from build123d import *

# Parameters (mm, degrees)
SKETCH1_W           = 36
SKETCH1_H           = 36
BOSS_EXTRUDE1_DEPTH = 186.9
FILLET1_SIZE        = 24
SKETCH2_R           = 2
CUT_EXTRUDE1_DEPTH  = 5
SKETCH3_W           = 4.8
SKETCH3_H           = 4.8
BOSS_EXTRUDE2_DEPTH = 4
SKETCH4_W           = 6
SKETCH4_H           = 4
CUT_EXTRUDE2_DEPTH  = 9
SKETCH5_W           = 3
SKETCH5_H           = 3
SKETCH5_W_2         = 12
SKETCH5_H_2         = 12
CUT_EXTRUDE3_DEPTH  = 10
SKETCH6_W           = 9
SKETCH6_H           = 6
CUT_EXTRUDE4_DEPTH  = 2


with BuildPart() as part:
    # Sketch1 → Boss-Extrude1 (new body)
    with BuildSketch(Plane(origin=(0, 0, 0), x_dir=(1, 0, 0), z_dir=(0, 1, 0))):
        with Locations((18, 18)):
            Rectangle(SKETCH1_W, SKETCH1_H)
    extrude(amount=BOSS_EXTRUDE1_DEPTH)

    # Fillet1
    # a fillet whose section is not a circle: 24 mm, written as the material it takes off along each edge
    with BuildSketch(Plane(origin=(0, -60, 0), x_dir=(1, 0, 0), z_dir=(0, 1, 0))) as fillet1_piece_1:
        with BuildLine():
            Bezier((FILLET1_SIZE, 0), (0, 0), (0, FILLET1_SIZE), weights=[1, 1.222222222, 1])
            Line((0, FILLET1_SIZE), (0, 0))
            Line((0, 0), (FILLET1_SIZE, 0))
        make_face()
    extrude(amount=306.9, mode=Mode.SUBTRACT)

    # Sketch2 → Cut-Extrude1 (cut)
    with BuildSketch(Plane.XZ):
        with Locations(Location((18, -18, 0), (0, 0, 270))):
            Circle(SKETCH2_R)
    extrude(amount=-CUT_EXTRUDE1_DEPTH, mode=Mode.SUBTRACT)

    # Sketch3 → Boss-Extrude2 (add)
    with BuildSketch(Plane.XZ):
        Polygon((26.2, -5), (31, -5), (31, -31), (26, -31), (5, -31), (5, -26.2), (26.2, -26.2), align=None)
        with Locations((11.8, -11.8)):
            Rectangle(SKETCH3_W, SKETCH3_H)
    extrude(amount=BOSS_EXTRUDE2_DEPTH)

    # Sketch4 → Cut-Extrude2 (cut)
    with BuildSketch(Plane(origin=(0, 0, -36), x_dir=(-1, 0, 0), z_dir=(0, 0, -1))):
        with Locations((-7, 180.9)):
            Rectangle(SKETCH4_W, SKETCH4_H)
        with Locations((-29, 180.9)):
            Rectangle(SKETCH4_W, SKETCH4_H)
        with Locations((-7, 160.9)):
            Rectangle(SKETCH4_W, SKETCH4_H)
    extrude(amount=-CUT_EXTRUDE2_DEPTH, mode=Mode.SUBTRACT)

    # Sketch5 → Cut-Extrude3 (cut)
    with BuildSketch(Plane(origin=(0, 186.9, 0), x_dir=(1, 0, 0), z_dir=(0, 1, 0))):
        with Locations((7, 31.5)):
            Rectangle(SKETCH5_W, SKETCH5_H)
        with Locations((18, 18)):
            Rectangle(SKETCH5_W_2, SKETCH5_H_2)
    extrude(amount=-CUT_EXTRUDE3_DEPTH, mode=Mode.SUBTRACT)

    # Sketch6 → Cut-Extrude4 (cut)
    with BuildSketch(Plane(origin=(0, 186.9, 0), x_dir=(1, 0, 0), z_dir=(0, 1, 0))):
        with Locations((7, 30)):
            Rectangle(SKETCH6_W, SKETCH6_H)
    extrude(amount=-CUT_EXTRUDE4_DEPTH, mode=Mode.SUBTRACT)


solid = part.part
Work out the finished part from the listing and answer in its coordinate system (mm). A direction names the side the tool comes from. Give positions to 0.01 mm unless a question says otherwise; leave off trailing zeros. Answer in a Markdown table with one row per item. Add a question column.
Q1. Determine the mould class of faces 1 (the flat face through (10, 181, -32)), 2 (the cylindrical face through (20, 2, -18)), 3 (the flat face through (12, -2, -9.4)) for opening direction Z: released by +Z, released by -Z, zero draft, split by the parting line, or undercut.
Q2. Consider line 1 along X through (y, z) = (177.5, -22); line 2 along Y through (x, z) = (33, -5); line 3 along X through (y, z) = (87, -22). Determine where each line is inside the solid, lowest interval first.
Q3. A tool of negligible diameter and unlimited length cuts with its end or side. For faces 4 (the flat face through (18, 182, -12)), 5 (the flat face through (26, 181, -32)), 6 (the flat face through (31, -2, -18)), 7 (the flat face through (9.4, -2, -12)), from which of +Z, -Z, +X, -X, +Y, -Y can it reach the whole face along a straight path? Write none if from no direction.
Q4. Each of these flat-tipped pins is pushed along its axis until it touches: P1, Ø4, axis at x = 24, y = 126, coming from the +Z side; P2, Ø2, axis at x = 28, y = -2, coming from the +Z side; P3, Ø2, axis at x = 11, y = -1.5, coming from the -Z side; P4, Ø1.2, axis at y = -1.5, z = -19.5, coming from the +X side. Where does it stop, or does it pass through?
Solution:
| question | item | result |
|---|---|---|
| 1 | face 1 | zero draft |
| 1 | face 2 | undercut |
| 1 | face 3 | released by +Z |
| 2 | line 1 | x = 0.03 to 12, 24 to 36 |
| 2 | line 2 | y = 0 to 186.9 |
| 2 | line 3 | x = 0.03 to 36 |
| 3 | face 4 | +Y |
| 3 | face 5 | -Z |
| 3 | face 6 | +Z, -Z, +X, -Y |
| 3 | face 7 | +Z, -X, -Y |
| 4 | P1 | stops at z = 0 |
| 4 | P2 | stops at z = -5 |
| 4 | P3 | stops at z = -31 |
| 4 | P4 | stops at x = 31 |
